Work out the finished part from the listing and answer in its coordinate system (mm). Face numbers are marked on the shaded views. A direction names the side the tool comes from. Round coordinates to 2 decimals unless told otherwise and drop trailing zeros. Write each loop counter-clockwise with the first axis right and the second up, starting at its lowest first coordinate (ties: lowest second). Pieces come first, ordered by that corner, then holes. Notation, with made-up numbers: (-35.5, 9.5) -> (11.5, 9.5) arc R22 cw to (11.5, 20.5) -> close; hole circle Ø7 at (40, -21.5). An arc over 180 degrees is marked (long way). One line per item, written item: value.
```python
from build123d import *

# Parameters (mm, degrees)
SKETCH_1_R          = 10
EXTRUDE_1_DEPTH     = 14
CUT_EXTRUDE_1_DEPTH = 500
SKETCH_4_R          = 8
CUT_EXTRUDE_2_DEPTH = 1000
SKETCH_6_R          = 10
EXTRUDE_2_DEPTH     = 1
SKETCH_5_R          = 2.000000000000003
EXTRUDE_3_DEPTH     = 7
SKETCH_5_2_R        = 2.000000000000003
CUT_EXTRUDE_3_DEPTH = 6
SKETCH_7_W          = 0.9999999999999662
SKETCH_7_H          = 12
EXTRUDE_4_DEPTH     = 5
EXTRUDE_5_DEPTH     = 12
SKETCH_9_W          = 12.6666666666667
SKETCH_9_H          = 12
CUT_EXTRUDE_4_DEPTH = 5
SKETCH_10_R         = 4
EXTRUDE_6_DEPTH     = 2
SKETCH_11_R         = 7
EXTRUDE_7_DEPTH     = 1
FILLET_1_R          = 3
FILLET_2_R          = 1
FILLET_4_R          = 1


with BuildPart() as part:
    # 草图1 → 凸台-拉伸1 (new body)
    with BuildSketch(Plane.XY):
        Circle(SKETCH_1_R)
    extrude(amount=EXTRUDE_1_DEPTH)

    # 草图3 → 切除-拉伸1 (cut, symmetric)
    with BuildSketch(Plane(origin=(0, 0, 0), x_dir=(1, 0, 0), z_dir=(0, 1, 0))):
        Polygon((-7.999999999999998, 0), (10, 0), (10, -12), align=None)
    extrude(amount=CUT_EXTRUDE_1_DEPTH, both=True, mode=Mode.SUBTRACT)

    # 草图4 → 切除-拉伸2 (cut)
    with BuildSketch(Plane.XY.offset(14)):
        Circle(SKETCH_4_R)
    extrude(amount=-CUT_EXTRUDE_2_DEPTH, mode=Mode.SUBTRACT)

    # 草图6 → 凸台-拉伸2 (add)
    with BuildSketch(Plane.XY.offset(14)):
        Circle(SKETCH_6_R)
    extrude(amount=EXTRUDE_2_DEPTH)

    # 草图5 → 凸台-拉伸3 (add, symmetric)
    with BuildSketch(Plane(origin=(0, 0, 0), x_dir=(1, 0, 0), z_dir=(0, 1, 0))):
        with BuildLine():
            Line((-5.9999999999999964, -14.999999999999968), (-11.999999999999996, -14.999999999999968))
            Line((-11.999999999999996, -14.999999999999968), (-17.71032629227648, -0.0718206378086078))
            ThreePointArc((-17.71032629227648, -0.0718206378086078), (-16.78084089382489, 3.3438624943348247), (-13.244226324520296, 3.496150883013566))
            Line((-13.244226324520296, 3.496150883013566), (-5.999999999999997, -1.333333333333298))
            Line((-5.999999999999997, -1.333333333333298), (-5.9999999999999964, -14.999999999999968))
        make_face()
        with Locations(Location((-14.908326913195987, 1.0000000000000329, 0), (0, 0, 270))):
            Circle(SKETCH_5_R, mode=Mode.SUBTRACT)
    extrude(amount=EXTRUDE_3_DEPTH, both=True)

    # 草图5<2> → 切除-拉伸3 (cut, symmetric)
    with BuildSketch(Plane(origin=(0, 0, 0), x_dir=(1, 0, 0), z_dir=(0, 1, 0))):
        with BuildLine():
            Line((-5.9999999999999964, -14.999999999999968), (-11.999999999999996, -14.999999999999968))
            Line((-11.999999999999996, -14.999999999999968), (-17.71032629227648, -0.0718206378086078))
            ThreePointArc((-17.71032629227648, -0.0718206378086078), (-16.78084089382489, 3.3438624943348247), (-13.244226324520296, 3.496150883013566))
            Line((-13.244226324520296, 3.496150883013566), (-5.999999999999997, -1.333333333333298))
            Line((-5.999999999999997, -1.333333333333298), (-5.9999999999999964, -14.999999999999968))
        make_face()
        with Locations(Location((-14.908326913195987, 1.0000000000000329, 0), (0, 0, 270))):
            Circle(SKETCH_5_2_R, mode=Mode.SUBTRACT)
    extrude(amount=CUT_EXTRUDE_3_DEPTH, both=True, mode=Mode.SUBTRACT)

    # 草图7 → 凸台-拉伸4 (add)
    with BuildSketch(Plane.ZY.offset(5.999999999999997)):
        with Locations((14.499999999999986, 0)):
            Rectangle(SKETCH_7_W, SKETCH_7_H)
    extrude(amount=EXTRUDE_4_DEPTH)

    # 草图8 → 凸台-拉伸5 (add)
    with BuildSketch(Plane.XZ.offset(-6)):
        Polygon((-11.999999999999996, 14.999999999999968), (-12.382519941228653, 14), (-10.999999999999996, 14), (-10.999999999999996, 14.999999999999968), align=None)
    extrude(amount=EXTRUDE_5_DEPTH)

    # 草图9 → 切除-拉伸4 (cut)
    with BuildSketch(Plane.ZY.offset(5.999999999999997)):
        with Locations((7.6666666666666465, 0)):
            Rectangle(SKETCH_9_W, SKETCH_9_H)
    extrude(amount=-CUT_EXTRUDE_4_DEPTH, mode=Mode.SUBTRACT)

    # 草图10 → 凸台-拉伸6 (add)
    with BuildSketch(Plane.XY.offset(15)):
        Circle(SKETCH_10_R)
    extrude(amount=EXTRUDE_6_DEPTH)

    # 草图11 → 凸台-拉伸7 (add)
    with BuildSketch(Plane.XY.offset(17)):
        Circle(SKETCH_11_R)
    extrude(amount=-EXTRUDE_7_DEPTH)

    # 圆角1
    fillet_1_edges = [part.edges().sort_by_distance(p)[0] for p in [
        (-5.291502622129181, -6, 7.902832459290273),
        (-5.291502622129181, 6, 7.902832459290272),
        (-7.14142842854285, -7, 7.7861905238190845),
        (-7.14142842854285, 7, 7.786190523819085),
    ]]
    fillet(fillet_1_edges, radius=FILLET_1_R)

    # 圆角2
    fillet_2_edges = [part.edges().sort_by_distance(p)[0] for p in [
        (-7, 8.6e-16, 16),
    ]]
    fillet(fillet_2_edges, radius=FILLET_2_R - 0.0001)  # a hair under: the kernel refuses the full size

    # 圆角4
    fillet_4_edges = [part.edges().sort_by_distance(p)[0] for p in [
        (10, -1.78e-15, 15),
        (-7.287574532187941, -7.178380170622118, 14.999999999999968),
        (-7.287574532187943, 7.178380170622118, 14.999999999999968),
        (-10.153311931459037, 7, 14.999999999999968),
        (-10.153311931459037, -7, 14.999999999999968),
    ]]
    fillet(fillet_4_edges, radius=FILLET_4_R)


solid = part.part
```
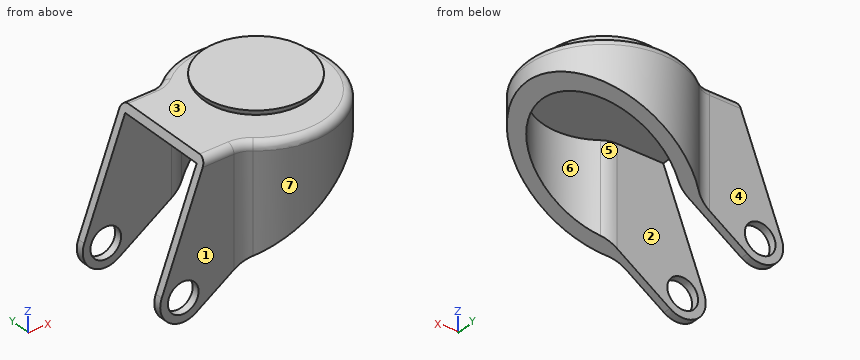
(1) A tool of negligible diameter and unlimited length cuts with its end or side. For the marked faces 1, 2 and 3, from which of +Z, -Z, +X, -X, +Y, -Y can it reach the whole face along a straight path? Write none if from no direction.
Reported:
face 1: +Z, -Z, -X, -Y
face 2: -Z, -X
face 3: none
(2) Flat-ended cylindrical pins translate along their axes: pin 1 Ø4.5 at (x, z) = (-14.91, -1) entering from -Y; pin 2 Ø3 at (x, z) = (-14.91, -1) entering from +Y; pin 3 Ø5 at (x, z) = (-7.5, 5) entering from -Y; pin 4 Ø3.5 at (x, z) = (-11.5, 3) entering from +Y. Find the tip coordinate at first contact, or state that the pin passes through.
Reported:
pin 1: stops at y = -7
pin 2: passes through
pin 3: stops at y = -8.66
pin 4: stops at y = 7
(3) For a pull along Y with two mould halves and no side action, classify the marked faces 4, 5, 6 and 7 as pulls with the +Y half, pulls with the -Y half, needs draft (parallel to the pull), parting line crosses it, or undercut.
Reported:
face 4: pulls with the +Y half
face 5: undercut
face 6: undercut
face 7: parting line crosses it
(4) Consider probe 1 along X at (y, z) = (6.25, -1); probe 2 along Z at (x, y) = (3.5, 5); probe 3 along Y at (x, z) = (-5, 8.5). Determine where each line is inside the solid, lowest interval first.
Reported:
probe 1: x = -17.91 to -16.91, -12.91 to -9.5
probe 2: z = 14 to 15, 16.01 to 17
probe 3: y = -8.66 to -6.31, 6.31 to 8.66
(5) Find section C-C on z = 3.75. Give the vertices of the cut face in (x, y) (3 decimals), plus the area to 3 significant figures.
Reported:
outline: (-16.303, -7) -> (-8.307, -7) arc R3 cw to (-6.39, -7.692) arc R10 ccw to (-2.375, -9.714) -> (-2.375, -7.639) arc R8 cw to (-4.6, -6.545) arc R3 ccw to (-6.325, -6) -> (-16.303, -6) -> close; (-16.303, 6) -> (-6.325, 6) arc R3 ccw to (-4.6, 6.545) arc R8 cw to (-2.375, 7.639) -> (-2.375, 9.714) arc R10 ccw to (-6.39, 7.692) arc R3 cw to (-8.307, 7) -> (-16.303, 7) -> close
area: 38.1 mm2
(6) Find section A-A on z = -1. Give the vertices of the cut face in (x, y), plus the area to 3 significant figures.
Reported:
outline: (-17.91, -7) -> (-16.91, -7) -> (-16.91, -6) -> (-17.91, -6) -> close; (-17.91, 6) -> (-16.91, 6) -> (-16.91, 7) -> (-17.91, 7) -> close; (-12.91, -7) -> (-9.5, -7) -> (-9.5, -6) -> (-12.91, -6) -> close; (-12.91, 6) -> (-9.5, 6) -> (-9.5, 7) -> (-12.91, 7) -> close
area: 8.82 mm2
(7) Find section B-B on x = -11. Give the vertices of the cut face in (y, z), plus the area to 3 significant figures.
Reported:
outline: (-7, -2) -> (-6, -2) -> (-6, 14) -> (6, 14) -> (6, -2) -> (7, -2) -> (7, 14) arc R1 ccw to (6, 15) -> (-6, 15) arc R1 ccw to (-7, 14) -> close
area: 45.6 mm2
